The listing builds one solid part. Answer for the finished solid, in the listing's coordinates (mm). Face numbers are marked on the shaded views. Round coordinates to 2 decimals unless told otherwise and drop trailing zeros. Loops run counter-clockwise (first coordinate to the right, second up) from the corner with the lowest first, then second, coordinate; pieces in that order, holes last. Notation, with made-up numbers: (24, 38) - (40, 38) arc R9 cw to (40, 49) - close; hole circle Ø7 at (-13.75, 17.25). An arc over 180 degrees is marked (long way). One line per item, written item: value.
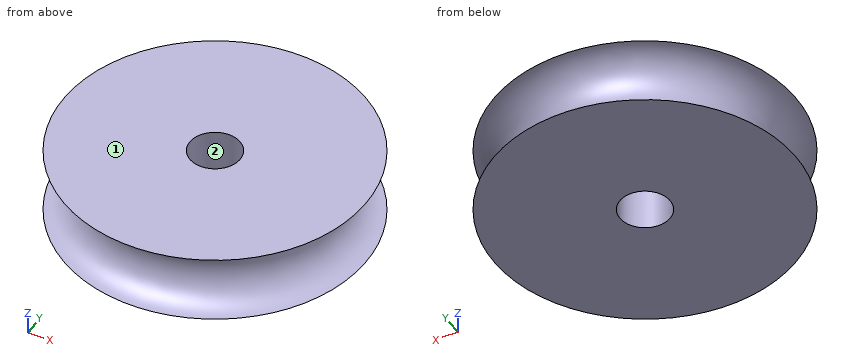
```python
from build123d import *

# Parameters (mm, degrees)
CYLINDER001_R     = 1.5
CYLINDER001_DEPTH = 5
TORUS_R           = 2
CYLINDER_R        = 9
CYLINDER_DEPTH    = 4


with BuildPart() as cylinder001:
    # Cylinder001 → Cylinder001 (new body)
    with BuildSketch(Plane.XY):
        Circle(CYLINDER001_R)
    extrude(amount=CYLINDER001_DEPTH)


with BuildPart() as torus:
    # Torus → Torus (revolve)
    with BuildSketch(Plane(origin=(0, 0, 2), x_dir=(1, 0, 0), z_dir=(0, -1, 0))):
        with Locations((9, 0)):
            Circle(TORUS_R)
    revolve(axis=Axis((0, 0, 2), (0, 0, 1)))


with BuildPart() as cut001:
    # Cylinder → Cylinder (new body)
    with BuildSketch(Plane.XY):
        Circle(CYLINDER_R)
    extrude(amount=CYLINDER_DEPTH)

    # Cut: cut Torus
    add(torus.part, mode=Mode.SUBTRACT)

    # Cut001: cut Cylinder001
    add(cylinder001.part, mode=Mode.SUBTRACT)


solid = cut001.part
```
1) A cutting plane is placed at A-A on x = 0. Give the vertices of the cut face in (y, z).
Final values:
outline: (-9, 0) - (-1.5, 0) - (-1.5, 4) - (-9, 4) arc R2 cw to start; (1.5, 0) - (9, 0) arc R2 cw to (9, 4) - (1.5, 4) - close
2) A cutting plane is placed at C-C on z = 2.55. Give the vertices of the cut face in (x, y).
Final values:
outline: circle Ø14.15 at (0, 0); hole circle Ø3 at (0, 0)
3) Consider L1, parallel to X at y = 0.5, z = 0.9; L2, parallel to Z at x = 7.25, y = -3.75; L3, parallel to X at y = 1.25, z = 3.15. Determine where each line is inside the solid, lowest interval first.
Final values:
L1: -7.31 to -1.41, 1.41 to 7.31
L2: 0 to 0.18, 3.82 to 4
L3: -7.26 to -0.83, 0.83 to 7.26
4) Each of these flat-tipped pins is pushed along its axis until it touches: pin 1 Ø1.5 at (x, z) = (-7, 2.5) entering from +Y; pin 2 Ø1.5 at (x, z) = (-3, 2.5) entering from -Y. Where does it stop, or does it pass through?
Final values:
pin 1: y = 3.4
pin 2: y = -6.88
5) For a pull along X with two mould halves and no side action, classify the marked faces 1 and 2 as released by +X, released by -X, zero draft, split by the parting line, or undercut.
Final values:
face 1: zero draft
face 2: undercut
